Geometry: final body of the model. Coordinates: model frame, mm. A direction names the side the tool comes from. Round coordinates to 2 decimals unless told otherwise and drop trailing zeros. Loops run counter-clockwise (first coordinate to the right, second up) from the corner with the lowest first, then second, coordinate; pieces in that order, holes last. Notation, with made-up numbers: M 48,-14.5 L 67,-14.5 A20 cw 67,-10.5 Z; hole C -37.75,43.25 d10. An arc over 180 degrees is marked long. Answer as a JSON object with one key per item and string values.
Autodesk Inventor part; units mm, degrees
ref_plane "YZ Plane" through (0, 0, 0) normal (1, 0, 0) x (0, 1, 0)
ref_plane "XZ Plane" through (0, 0, 0) normal (0, 1, 0) x (-1, 0, 0)
ref_plane "XY Plane" through (0, 0, 0) normal (0, 0, 1) x (1, 0, 0)
sketch "Sketch1" plane through (0, 0, 0) normal (0, 0, 1) x (1, 0, 0)
  line L0 (-42.6611, 7.6335) -> (42.1293, 7.6335) construction
  line L1 (25.6024, 7.6335) -> (25.6024, 17.6335)
  line L2 (25.6024, 17.6335) -> (20.6024, 17.6335)
  line L3 (20.6024, 17.6335) -> (20.6024, 15.6335)
  line L4 (20.6024, 15.6335) -> (15.6024, 15.6335)
  line L5 (15.6024, 15.6335) -> (15.6024, 13.6335)
  line L6 (15.6024, 13.6335) -> (10.6024, 13.6335)
  line L7 (10.6024, 13.6335) -> (10.6024, 11.6335)
  line L8 (10.6024, 11.6335) -> (5.6024, 11.6335)
  line L9 (5.6024, 11.6335) -> (5.6024, 9.6335)
  line L10 (5.6024, 9.6335) -> (-0.3976, 9.6335)
  arc A0 (-0.3976, 9.6335) -> (-1.1976, 11.2335) centre (-1.1976, 10.2335) ccw
  line L11 (-1.1976, 10.2335) -> (-1.1976, 7.6335)
  line L12 (-1.1976, 10.2335) -> (-1.1976, 11.2335)
  line L13 (-1.1976, 7.6335) -> (25.6024, 7.6335)
  point P0 (0, 0)
  dimension "d2" = 5
  dimension "d3" = 5
  dimension "d4" = 5
  dimension "d5" = 5
  dimension "d7" = 2
  dimension "d8" = 2
  dimension "d9" = 2
  dimension "d10" = 2
  dimension "d11" = 2
  dimension "d12" = 2
revolve "Revolution1" add sketch "Sketch1" angle 360 about axis through (-42.6611, 7.6335, 0) along (1, 0, 0)
properties part number "lesson4"
1) Line query: probe 1 along Y at (x, z) = (23, 0.25); probe 2 along X at (y, z) = (11, -8.75); probe 3 along X at (y, z) = (10.25, 5). Output: solid intervals per line, ascending.
Geometry results:
{"probe 1": "-2.36 to 17.63", "probe 2": "20.6 to 25.6", "probe 3": "10.6 to 25.6"}
2) Cut plane D-D on z = 5.5. Return the cut outline in (x, y).
Geometry results:
{"outline": "M 10.6,5.24 L 15.6,5.24 L 15.6,1.82 L 20.6,1.82 L 20.6,-0.72 L 25.6,-0.72 L 25.6,15.99 L 20.6,15.99 L 20.6,13.44 L 15.6,13.44 L 15.6,10.03 L 10.6,10.03 Z"}
3) Cut plane A-A on z = 0. Return the cut outline in (x, y).
Geometry results:
{"outline": "M -1.2,4.03 A1 ccw -0.4,5.63 L 5.6,5.63 L 5.6,3.63 L 10.6,3.63 L 10.6,1.63 L 15.6,1.63 L 15.6,-0.37 L 20.6,-0.37 L 20.6,-2.37 L 25.6,-2.37 L 25.6,17.63 L 20.6,17.63 L 20.6,15.63 L 15.6,15.63 L 15.6,13.63 L 10.6,13.63 L 10.6,11.63 L 5.6,11.63 L 5.6,9.63 L -0.4,9.63 A1 ccw -1.2,11.23 Z"}
4) Pull-direction query (X, two-part tool) for faces 1 (the face through (18.07, 5.9, 7.81)), 2 (the face through (15.602, 9, 6)), 3 (the face through (2.56, 7.2, 1.952)), 4 (the face through (5.602, 9, -2)); classes: +X half, -X half, draft (parallel to the pull), parting line (faces both ways), or undercut.
Geometry results:
{"face 1": "draft", "face 2": "-X half", "face 3": "undercut", "face 4": "undercut"}
5) First-contact query: pin 1 (12 mm diameter, centred on x = 11.5, z = -4.5, fed in from +Y); pin 2 (2 mm diameter, centred on x = 22, z = -7.5, fed in from +Y); pin 3 (1 mm diameter, centred on x = 9.5, y = 4.5, fed in from +Z). Flat tips, straight axial feed; report the tip coordinate or a pass-through.
Geometry results:
{"pin 1": "y = 15.63", "pin 2": "y = 15.23", "pin 3": "z = 3.01"}
6) Cut plane C-C on z = 7.5. Return the cut outline in (x, y).
Geometry results:
{"outline": "M 15.6,4.85 L 20.6,4.85 L 20.6,1.02 L 25.6,1.02 L 25.6,14.25 L 20.6,14.25 L 20.6,10.42 L 15.6,10.42 Z"}
7) Cut plane B-B on x = 3.25. Return the cut outline in (y, z).
Geometry results:
{"outline": "C 7.63,0 d4"}
8) Set-up query: faces 5 (the face through (25.602, 7, 0)), 6 (the face through (8.07, 11.33, 1.53)). Return all of +Z, -Z, +X, -X, +Y, -Y with unobstructed straight access to the full face (end or side cutting, diameter ignored); none if empty.
Geometry results:
{"face 5": "+Z, -Z, +X, +Y, -Y", "face 6": "-X"}
